The listing builds one solid part. Answer for the finished solid, in the listing's coordinates (mm). Coordinates: 2 decimals unless noted, no trailing zeros. Loops run counter-clockwise (first coordinate to the right, second up) from the corner with the lowest first, then second, coordinate; pieces in that order, holes last. Notation, with made-up numbers: (45, 18.25) - (70, 18.25) arc R19 ccw to (70, 52.25) - close; hole circle Ø3 at (-33.75, -21.5). An arc over 180 degrees is marked (long way). Return JSON: item names as keys, results as strings. Group by question number.
1. Section B-B (y = 3.75) is taken. Write down the section's boundary in (x, z), and give its area (3 significant figures).
2. Section A-A (x = 33.5) is taken. Write down the section's boundary in (y, z), and give its area (3 significant figures).
3. Find the intervals of material crossed by line 1 along Z through (x, y) = (-33, 4.75); line 2 along X through (y, z) = (2.75, 28.5), in increasing order.
4. Section C-C (z = 23.5) is taken. Write down the section's boundary in (x, y), and give its area (3 significant figures).
5. Each of these flat-tipped pins is pushed along its axis until it touches: P1, Ø1.9, axis at y = 3.5, z = 67.5, coming from the -X side; P2, Ø3, axis at x = -35, y = 4, coming from the +Z side; P3, Ø4, axis at x = -18, z = -45.5, coming from the -Y side. Where does it stop, or does it pass through?
```python
from build123d import *

# Parameters (mm, degrees)
SKETCH1_W           = 76.2
SKETCH1_H           = 127
BOSS_EXTRUDE1_DEPTH = 6.35
CAVITY1_START       = -38.1
CAVITY1_OUTLINE_W   = 6.35
CAVITY1_OUTLINE_H   = 25.4
CAVITY1_DEPTH       = 6.35
CAVITY1_START_2     = 31.75
CAVITY1_2_OUTLINE_W = 6.35
CAVITY1_2_OUTLINE_H = 25.4
CAVITY1_2_DEPTH     = 6.35
SKETCH2_W           = 63.5
SKETCH2_H           = 6.35
BOSS_EXTRUDE2_DEPTH = 6.35
SKETCH3_W           = 63.5
SKETCH3_H           = 6.35
BOSS_EXTRUDE3_DEPTH = 12.7


# Read off the part's stored shape, not the designer's step: Cavity1
with BuildPart() as part:
    # Sketch1 → Boss-Extrude1 (new body)
    with BuildSketch(Plane(origin=(0, 0, 0), x_dir=(1, 0, 0), z_dir=(0, 1, 0))):
        Rectangle(SKETCH1_W, SKETCH1_H)
    extrude(amount=BOSS_EXTRUDE1_DEPTH)

    # Cavity1 outline → Cavity1 (cut)
    with BuildSketch(Plane.YZ.offset(CAVITY1_START)):
        with Locations((3.175, 25.4)):
            Rectangle(CAVITY1_OUTLINE_W, CAVITY1_OUTLINE_H)
        with Locations((3.175, -25.4)):
            Rectangle(CAVITY1_OUTLINE_W, CAVITY1_OUTLINE_H)
    extrude(amount=CAVITY1_DEPTH, mode=Mode.SUBTRACT)

    # Cavity1 2 outline → Cavity1 2 (cut)
    with BuildSketch(Plane.YZ.offset(CAVITY1_START_2)):
        with Locations((3.175, 25.4)):
            Rectangle(CAVITY1_2_OUTLINE_W, CAVITY1_2_OUTLINE_H)
        with Locations((3.175, -25.4)):
            Rectangle(CAVITY1_2_OUTLINE_W, CAVITY1_2_OUTLINE_H)
    extrude(amount=CAVITY1_2_DEPTH, mode=Mode.SUBTRACT)

    # Sketch2 → Boss-Extrude2 (add)
    with BuildSketch(Plane.XY.offset(63.5)):
        with Locations((0, 3.175)):
            Rectangle(SKETCH2_W, SKETCH2_H)
    extrude(amount=BOSS_EXTRUDE2_DEPTH)

    # Sketch3 → Boss-Extrude3 (add)
    with BuildSketch(Plane(origin=(0, 0, -63.5), x_dir=(-1, 0, 0), z_dir=(0, 0, -1))):
        with Locations((0, 3.175)):
            Rectangle(SKETCH3_W, SKETCH3_H)
    extrude(amount=BOSS_EXTRUDE3_DEPTH)


solid = part.part
```
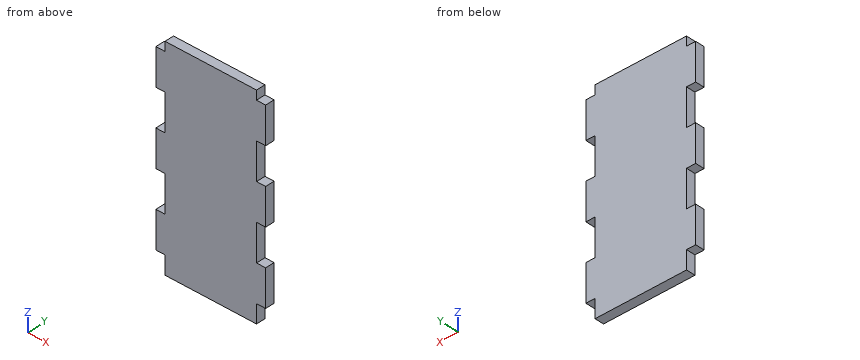
The answers:
{
 "1": {"outline": "(-38.1, -63.5) - (-31.75, -63.5) - (-31.75, -76.2) - (31.75, -76.2) - (31.75, -63.5) - (38.1, -63.5) - (38.1, -38.1) - (31.75, -38.1) - (31.75, -12.7) - (38.1, -12.7) - (38.1, 12.7) - (31.75, 12.7) - (31.75, 38.1) - (38.1, 38.1) - (38.1, 63.5) - (31.75, 63.5) - (31.75, 69.85) - (-31.75, 69.85) - (-31.75, 63.5) - (-38.1, 63.5) - (-38.1, 38.1) - (-31.75, 38.1) - (-31.75, 12.7) - (-38.1, 12.7) - (-38.1, -12.7) - (-31.75, -12.7) - (-31.75, -38.1) - (-38.1, -38.1) - close", "area": "10,200 mm2"},
 "2": {"outline": "(0, -63.5) - (6.35, -63.5) - (6.35, -38.1) - (0, -38.1) - close; (0, -12.7) - (6.35, -12.7) - (6.35, 12.7) - (0, 12.7) - close; (0, 38.1) - (6.35, 38.1) - (6.35, 63.5) - (0, 63.5) - close", "area": "484 mm2"},
 "3": {"line 1": "z = -63.5 to -38.1, -12.7 to 12.7, 38.1 to 63.5", "line 2": "x = -31.75 to 31.75"},
 "4": {"outline": "(-31.75, 0) - (31.75, 0) - (31.75, 6.35) - (-31.75, 6.35) - close", "area": "403 mm2"},
 "5": {"P1": "stops at x = -31.75", "P2": "stops at z = 63.5", "P3": "stops at y = 0"}
}
